Here's the drawing with two shaded views (mm, measured from the low corner). I have some questions. Coordinates: 2 decimals unless noted, no trailing zeros. Write each loop counter-clockwise with the first axis right and the second up, starting at its lowest first coordinate (ties: lowest second). Pieces come first, ordered by that corner, then holes.
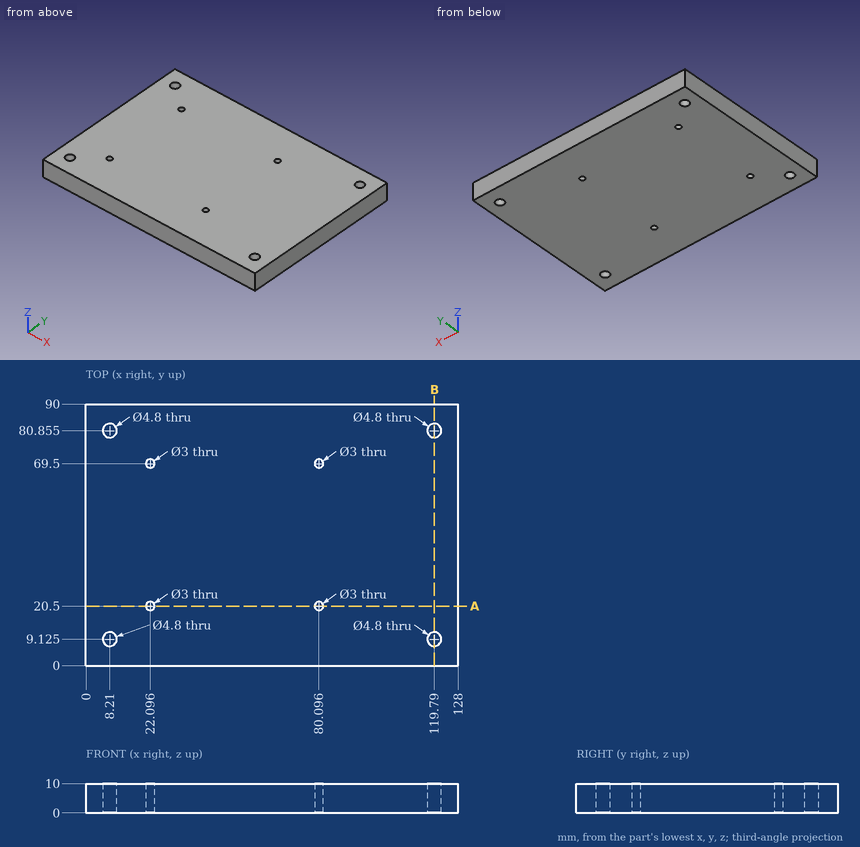
1. If we section it at A-A, the plane y = 20.5: List the corners of the cut face in (x, z) for me (1 decimal), plus the area to 3 significant figures.
2. I'm going to push a flat-ended pin straight in: P1, Ø4.5, axis at x = 8.21, y = 80.855, coming from the -Z side. Where does the tip first touch, or does it pass through?
3. If I drill on L1, parallel to X at y = 69.5, z = 7 (1 decimal); L2, parallel to Y at x = 8.21, z = 7.5 (1 decimal); L3, parallel to Y at x = 8.5, z = 7.25, over which ranges is the centre line in solid material (lowest first)?
4. If we section it at B-B, the plane x = 119.79: List the corners of the cut face in (y, z) for me (1 decimal), plus the area to 3 significant figures.
Answers:
1. outline: (0, 0) - (20.6, 0) - (20.6, 10) - (0, 10) - close; (23.6, 0) - (78.6, 0) - (78.6, 10) - (23.6, 10) - close; (81.6, 0) - (128, 0) - (128, 10) - (81.6, 10) - close
1. area: 1,220 mm2
2. P1: passes through
3. L1: x = 0 to 20.6, 23.6 to 78.6, 81.6 to 128
3. L2: y = 0 to 6.7, 11.5 to 78.5, 83.3 to 90
3. L3: y = 0 to 6.74, 11.51 to 78.47, 83.24 to 90
4. outline: (0, 0) - (6.7, 0) - (6.7, 10) - (0, 10) - close; (11.5, 0) - (78.5, 0) - (78.5, 10) - (11.5, 10) - close; (83.3, 0) - (90, 0) - (90, 10) - (83.3, 10) - close
4. area: 804 mm2
